Design review of the part built by this model. Coordinates are the model's own, in mm. A direction names the side the tool comes from. Give positions to 0.01 mm unless a question says otherwise; leave off trailing zeros. Order: outer loops, then holes, each group sorted by start corner. A loop starts at its lowest first (then second) coordinate and runs counter-clockwise, first axis right, second up. Notation, with made-up numbers: (-22, 87) -> (-14, 87) arc R32 ccw to (-14, 124) -> close; hole circle Ø1 at (17.5, -40). An arc over 180 degrees is marked (long way). Use a Markdown table: item, result. Add a question column.
```python
from build123d import *

# Parameters (mm, degrees)
F1_DEPTH = 3.175
F2_W     = 22.225
F2_H     = 3.175
F2_W_2   = 3.175
F2_H_2   = 22.225
F3_DEPTH = 25.4


with BuildPart() as f1:
    # F0 (on Front) → F1 (new body)
    with BuildSketch(Plane.XZ):
        with BuildLine():
            Line((-60.325, 0), (0, 0))
            Line((0, 0), (0, 60.325))
            ThreePointArc((0, 60.325), (-42.656217, 42.656217), (-60.325, 0))
        make_face()
    extrude(amount=F1_DEPTH)

    # F2 (on face) → F3 (cut)
    with BuildSketch(Plane.XZ.offset(3.175)):
        with Locations((-49.2125, 1.5875)):
            Rectangle(F2_W, F2_H)
        with Locations((-1.5875, 1.5875)):
            Rectangle(F2_W_2, F2_H)
        with Locations((-14.2875, 1.5875)):
            Rectangle(F2_W, F2_H)
        with Locations((-1.5875, 14.2875)):
            Rectangle(F2_W_2, F2_H_2)
        with Locations((-1.5875, 49.2125)):
            Rectangle(F2_W_2, F2_H_2)
        Polygon((0, 29.845), (0, 31.75), (0, 33.655), (-3.81, 33.655), (-3.81, 31.75), (-3.81, 29.845), align=None)
        Polygon((-33.655, 0), (-31.75, 0), (-29.845, 0), (-29.845, 3.81), (-31.75, 3.81), (-33.655, 3.81), align=None)
    extrude(amount=-F3_DEPTH, mode=Mode.SUBTRACT)


solid = f1.part
```
1) Machinability: for faces 4 (the flat face through (-2, -2, 25.4)), 5 (the flat face through (-49, -2, 3.175)), 6 (the flat face through (-29.845, -2, 2)), 7 (the flat face through (-3.175, -2, 49)), 8 (the flat face through (-2, -2, 29.845)), which of the approach directions +Z, -Z, +X, -X, +Y, -Y give a long, thin tool a straight path to every point of the face, cutting with its end or side? Answer none if there is none.
2) Add section C-C (x = -44). Give the boundary of the cut face in (y, z) (3 decimals).
3) Add section A-A (y = -1.9). Give the boundary of the cut face in (x, z) (3 decimals), then the cut area to 3 significant figures.
4) Insertion check: pin 1 (1 mm diameter, centred on y = -1, z = 2, fed in from +X); pin 2 (1 mm diameter, centred on x = -17.5, y = -1, fed in from -Z) (3 decimals); pin 3 (1 mm diameter, centred on x = -32, y = -2, fed in from -Z). Each pin has a flat end and moves straight along its axis. Give the tip position at first contact, or say it passes through.
5) Add section B-B (z = 22). Give the boundary of the cut face in (x, y) (3 decimals).
6) The part is to be moulded in two halves that separate along Z. For faces 1 (the flat face through (-36, -2, 0)), 2 (the flat face through (-2, -2, 33.655)), 3 (the flat face through (-24, -3.175, 24)), say which applies: +Z half, -Z half, draft (parallel to the pull), parting line (faces both ways), or undercut.
7) For L1, parallel to Z at x = -53, y = -0.3 (3 decimals); L2, parallel to Z at x = -45, y = -2.5 (3 decimals); L3, parallel to X at y = -0.45, z = 48 (3 decimals), list the stretches that pass through material, from the lowest coordinate up. Write a range as [from, to].
Worked answers:
| question | item | result |
|---|---|---|
| 1 | face 4 | -Z, +X, +Y, -Y |
| 1 | face 5 | -Z, -X, +Y, -Y |
| 1 | face 6 | -Z, +Y, -Y |
| 1 | face 7 | +Z, +X, +Y, -Y |
| 1 | face 8 | +X, +Y, -Y |
| 2 | outline | (-3.175, 3.175) -> (0, 3.175) -> (0, 41.269) -> (-3.175, 41.269) -> close |
| 3 | outline | (-60.241, 3.175) -> (-38.1, 3.175) -> (-38.1, 0) -> (-33.655, 0) -> (-33.655, 3.81) -> (-29.845, 3.81) -> (-29.845, 0) -> (-25.4, 0) -> (-25.4, 3.175) -> (-3.175, 3.175) -> (-3.175, 25.4) -> (0, 25.4) -> (0, 29.845) -> (-3.81, 29.845) -> (-3.81, 33.655) -> (0, 33.655) -> (0, 38.1) -> (-3.175, 38.1) -> (-3.175, 60.241) arc R60.325 ccw to start |
| 3 | area | 2,540 mm^2 |
| 4 | pin 1 | x = -25.4 |
| 4 | pin 2 | z = 3.175 |
| 4 | pin 3 | z = 3.81 |
| 5 | outline | (-56.17, -3.175) -> (-3.175, -3.175) -> (-3.175, 0) -> (-56.17, 0) -> close |
| 6 | face 1 | -Z half |
| 6 | face 2 | undercut |
| 6 | face 3 | draft |
| 7 | L1 | [3.175, 28.812] |
| 7 | L2 | [3.175, 40.176] |
| 7 | L3 | [-36.539, -3.175] |
